from build123d import *

# Parameters (mm, degrees)
ESQUISSE1_R                  = 156
BOSS_EXTRU_1_DEPTH           = 520
COQUE1_T                     = 3
ENL_V_MAT_EXTRU_1_DEPTH      = 565.864585542
ENL_V_MAT_EXTRU_1_DEPTH_BACK = 565.864585542
ESQUISSE3_W                  = 1
ESQUISSE3_H                  = 353.000816996
ENL_V_MAT_EXTRU_2_DEPTH      = 529.272656873


with BuildPart() as part:
    # Esquisse1 → Boss.-Extru.1 (new body)
    with BuildSketch(Plane(origin=(0, 0, 0), x_dir=(1, 0, 0), z_dir=(0, 1, 0))):
        with Locations(Location((0, 0, 0), (0, 0, 270))):
            Circle(ESQUISSE1_R)
    extrude(amount=BOSS_EXTRU_1_DEPTH)

    # Coque1 (no face opened: a closed hollow body)
    add(offset(amount=-COQUE1_T, mode=Mode.PRIVATE), mode=Mode.SUBTRACT)

    # Esquisse2 → Enlèv. mat.-Extru.1 (cut, two sides: drawn at the far end of the back side and taken through both)
    with BuildSketch(Plane.XY.offset(-ENL_V_MAT_EXTRU_1_DEPTH_BACK)):
        Polygon((0, 140), (-156.821895425, 140), (-156, 236), (0, 236), align=None)
        Polygon((-156, 520), (-156, 480), (26, 480), (156, 350), (156, 520), align=None)
    extrude(amount=ENL_V_MAT_EXTRU_1_DEPTH + ENL_V_MAT_EXTRU_1_DEPTH_BACK, mode=Mode.SUBTRACT)

    # Esquisse3 → Enlèv. mat.-Extru.2 (cut, through all)
    with BuildSketch(Plane(origin=(0, 0, 0), x_dir=(0, 0, -1), z_dir=(1, 0, 0))):
        with Locations((0, 176.500408498)):
            Rectangle(ESQUISSE3_W, ESQUISSE3_H)
    extrude(amount=ENL_V_MAT_EXTRU_2_DEPTH, mode=Mode.SUBTRACT)


solid = part.part
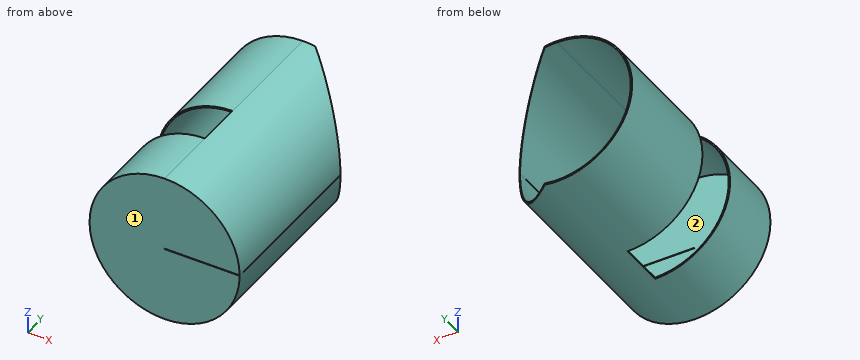
Design review of the part built by this model. Coordinates are the model's own, in mm. Face numbers are marked on the shaded views. Round coordinates to 2 decimals unless told otherwise and drop trailing zeros. Write each loop counter-clockwise with the first axis right and the second up, starting at its lowest first coordinate (ties: lowest second). Pieces come first, ordered by that corner, then holes. Notation, with made-up numbers: (-37.5, 78) - (-15.5, 78) arc R16 ccw to (-15.5, 102) - close; hole circle Ø7 at (55, 78). An arc over 180 degrees is marked (long way). Return JSON: item names as keys, results as strings. Group by question number.
Item 1: We need section B-B on x = -67. Write out the cut boundary in (y, z), and give its area (3 significant figures).
Item 2: We need section D-D on y = 66. Write out the cut boundary in (x, z).
Item 3: Insertion check: P1, Ø0.8, axis at y = 1, z = 0, coming from the +X side; P2, Ø2, axis at y = 252, z = 12.5, coming from the -X side; P3, Ø1.5, axis at x = 4, z = 50, coming from the +Y side. Each pin has a flat end and moves straight along its axis. Give the tip position at first contact, or say it passes through.
Item 4: The part is to be moulded in two halves that separate along X. For the marked faces 1 and 2, say which applies: pulls with the +X half, pulls with the -X half, needs draft (parallel to the pull), parting line crosses it, or undercut.
Item 5: For probe 1 along Z at (x, y) = (0, 351); probe 2 along Y at (x, z) = (-25, -19.5); probe 3 along Z at (x, y) = (80, 121), list the stretches that pass through material, from the lowest coordinate up. Write a range as [from, to].
Item 6: We need section A-A on z = 64.5. Write out the cut boundary in (x, y).
Item 7: We need section C-C on x = 36.5. Write out the cut boundary in (y, z), and give its area (3 significant figures).
Model answer:
{
 "1": {"outline": "(0, -140.88) - (140, -140.88) - (140, -137.55) - (3, -137.55) - (3, 137.55) - (140, 137.55) - (140, 140.88) - (0, 140.88) - close; (236, -140.88) - (480, -140.88) - (480, -137.55) - (236, -137.55) - close; (236, 137.55) - (480, 137.55) - (480, 140.88) - (236, 140.88) - close", "area": "3,380 mm²"},
 "2": {"outline": "(153, -0.5) arc R153 cw (long way) to (153, 0.5) - (156, 0.5) arc R156 ccw (long way) to (156, -0.5) - close"},
 "3": {"P1": "stops at x = 0", "P2": "stops at x = -155.58", "P3": "stops at y = 3"},
 "4": {"face 1": "needs draft", "face 2": "undercut"},
 "5": {"probe 1": "z = [-156, -153], [153, 156]", "probe 2": "y = [0, 3]", "probe 3": "z = [-133.93, -130.42], [130.42, 133.93]"},
 "6": {"outline": "(-142.04, 0) - (142.04, 0) - (142.04, 363.96) - (138.74, 367.26) - (138.74, 3) - (-138.74, 3) - (-138.74, 140) - (-142.04, 140) - close; (-142.04, 236) - (-138.74, 236) - (-138.74, 480) - (-142.04, 480) - close"},
 "7": {"outline": "(0, -151.67) - (469.5, -151.67) - (469.5, -148.58) - (3, -148.58) - (3, -0.5) - (0, -0.5) - close; (0, 0.5) - (3, 0.5) - (3, 148.58) - (469.5, 148.58) - (469.5, 151.67) - (0, 151.67) - close", "area": "3,790 mm²"}
}
